Answer from the drawing. Dimensions are ordinates in mm from the lowest x, y and z of the part. Coordinates: 2 decimals unless noted, no trailing zeros. Order: outer loops, then holes, each group sorted by start corner. A loop starts at its lowest first (then second) coordinate and runs counter-clockwise, first axis right, second up. Notation, with made-up numbers: (-22, -32) -> (21, -32) arc R28 ccw to (21, -1) -> close; hole circle Ø2 at (-15.5, -25.75). An arc over 180 degrees is marked (long way). Answer in a Markdown table with one row per item.
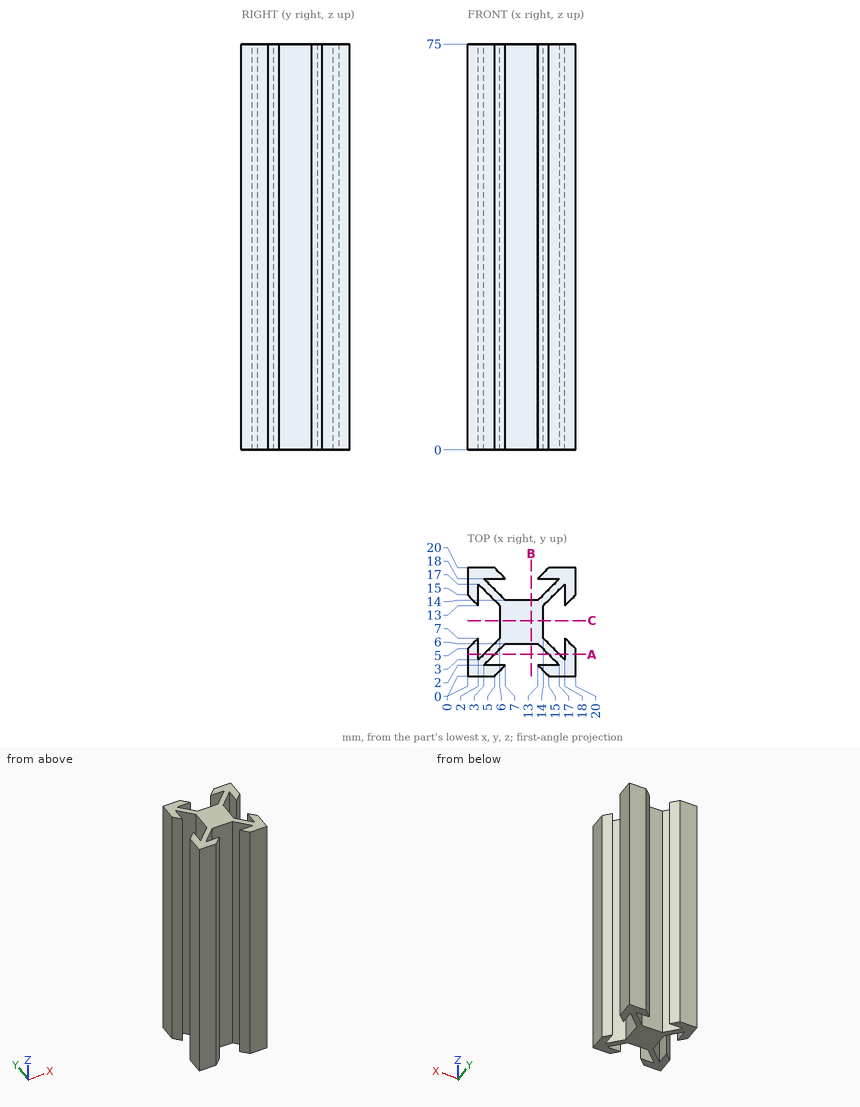
(1) Find the intervals of material crossed by line 1 along Y through (x, z) = (4.25, 59.5); line 2 along Y through (x, z) = (6.5, 51); line 3 along X through (y, z) = (16, 42.5), in increasing order. Write a range as from..to.
Check values:
| item | result |
|---|---|
| line 1 | 0..2, 3.25..5.25, 14.75..16.75, 18..20 |
| line 2 | 1.5..2, 5.5..14.5, 18..18.5 |
| line 3 | 0..2, 3..5, 15..17, 18..20 |
(2) A cutting plane is placed at A-A, the plane y = 4. Determine the outline of the cut face in (x, z).
Check values:
| item | result |
|---|---|
| outline | (0, 0) -> (2, 0) -> (2, 75) -> (0, 75) -> close; (3, 0) -> (5, 0) -> (5, 75) -> (3, 75) -> close; (15, 0) -> (17, 0) -> (17, 75) -> (15, 75) -> close; (18, 0) -> (20, 0) -> (20, 75) -> (18, 75) -> close |
(3) Flat-ended cylindrical pins translate along their axes: pin 1 (5 mm diameter, centred on y = 8.5, z = 34, fed in from -X); pin 2 (3 mm diameter, centred on x = 15, z = 38, fed in from -Y); pin 3 (1.8 mm diameter, centred on y = 11, z = 53, fed in from +X); pin 4 (3 mm diameter, centred on x = 9.5, z = 27.5, fed in from -Y). Find the tip coordinate at first contact, or state that the pin passes through.
Check values:
| item | result |
|---|---|
| pin 1 | x = 1 |
| pin 2 | y = 0 |
| pin 3 | x = 14 |
| pin 4 | y = 6 |
(4) A cutting plane is placed at B-B, the plane x = 11.75. Determine the outline of the cut face in (y, z).
Check values:
| item | result |
|---|---|
| outline | (6, 0) -> (14, 0) -> (14, 75) -> (6, 75) -> close |
